```python
from build123d import *

# Parameters (mm, degrees)
SKETCH1_W           = 5
SKETCH1_H           = 5
BOSS_EXTRUDE1_DEPTH = 40
SKETCH2_W           = 51.86
SKETCH2_H           = 5
SKETCH2_W_2         = 5
BOSS_EXTRUDE3_DEPTH = 5
SKETCH4_W           = 25
SKETCH4_H           = 5
BOSS_EXTRUDE4_DEPTH = 15
FILLET1_R           = 1
FILLET2_R           = 1
FILLET3_R           = 1
SKETCH5_W           = 10
SKETCH5_H           = 6
CUT_EXTRUDE1_DEPTH  = 70.699782068


with BuildPart() as part:
    # Sketch1 → Boss-Extrude1 (new body)
    with BuildSketch(Plane(origin=(0, 0, 0), x_dir=(1, 0, 0), z_dir=(0, 1, 0))):
        with Locations((2.5, 2.5)):
            Rectangle(SKETCH1_W, SKETCH1_H)
    extrude(amount=BOSS_EXTRUDE1_DEPTH)

    # Sketch2 → Boss-Extrude3 (add)
    with BuildSketch(Plane.XZ):
        with Locations((30.93, -2.5)):
            Rectangle(SKETCH2_W, SKETCH2_H)
        with Locations((2.5, -2.5)):
            Rectangle(SKETCH2_W_2, SKETCH2_H)
    extrude(amount=BOSS_EXTRUDE3_DEPTH)

    # Sketch4 → Boss-Extrude4 (add)
    with BuildSketch(Plane.XZ.offset(5)):
        with Locations((44.36, -2.5)):
            Rectangle(SKETCH4_W, SKETCH4_H)
    extrude(amount=BOSS_EXTRUDE4_DEPTH)

    # Fillet1
    fillet1_edges = [part.edges().sort_by_distance(p)[0] for p in [
        (15.93, -5, 0),
        (56.86, -10, 0),
        (30.93, 0, 0),
        (31.86, -12.5, 0),
        (44.36, -20, 0),
    ]]
    fillet(fillet1_edges, radius=FILLET1_R)

    # Fillet2
    fillet2_edges = [part.edges().sort_by_distance(p)[0] for p in [
        (56.86, -10, -5),
        (30.93, 0, -5),
        (15.93, -5, -5),
        (31.86, -12.5, -5),
        (44.36, -20, -5),
    ]]
    fillet(fillet2_edges, radius=FILLET2_R)

    # Fillet3
    fillet3_edges = [part.edges().sort_by_distance(p)[0] for p in [
        (5, 0, -2.5),
        (5, -0.292893219, -0.292893219),
        (5, -0.292893219, -4.707106781),
    ]]
    fillet(fillet3_edges, radius=FILLET3_R)

    # Sketch5 → Cut-Extrude1 (cut, through all)
    with BuildSketch(Plane(origin=(0, 0, -5), x_dir=(-1, 0, 0), z_dir=(0, 0, -1))):
        with Locations((-45.36, -6.38)):
            Rectangle(SKETCH5_W, SKETCH5_H)
    extrude(amount=-CUT_EXTRUDE1_DEPTH, mode=Mode.SUBTRACT)


solid = part.part
```
Check sheet for the modelled part. Datum: model origin and axes. Units: mm. A direction names the side the tool comes from. Give positions to 0.01 mm unless a question says otherwise; leave off trailing zeros. Write each loop counter-clockwise with the first axis right and the second up, starting at its lowest first coordinate (ties: lowest second). Pieces come first, ordered by that corner, then holes. Notation, with made-up numbers: (-31, 52.25) -> (26, 52.25) arc R27 ccw to (26, 73.25) -> close; hole circle Ø7 at (-31.75, 36). An arc over 180 degrees is marked (long way). Use CSV: the item, a comma, the result in double quotes. Start each with the question number.
Q1. Cross-section at B-B on x = 45. Enter the section's corners in (y, z).
Q2. Tool access check on faces 1 (the flat face through (50.36, -6, -3)), 2 (the flat face through (28, -2, 0)), 3 (the flat face through (31.86, -12, -3)), 4 (the flat face through (31, 0, -2)). Record the directions out of +Z, -Z, +X, -X, +Y, -Y that give a thin tool (end or side, any length) a straight path to the whole face; none if there is none.
Q3. Cross-section at C-C on x = 7. Enter the section's corners in (y, z), and give its area (3 significant figures).
Q4. Depth check by flat-ended pin: P1, Ø1.5, axis at x = 33.5, z = -2.5, coming from the +Y side; P2, Ø3, axis at x = 8, z = -1.5, coming from the -Y side; P3, Ø0.9, axis at y = -16, z = -2.5, coming from the -X side. Enter the tip coordinate at first touch or a pass-through.
Q5. Cross-section at D-D on y = 21.5. Enter the section's corners in (x, z).
Q6. Scan lines: line 1 along Y through (x, z) = (46, -3.1); line 2 along X through (y, z) = (9, -1.8); line 3 along Y through (x, z) = (53, -3.6). Record each from-to range of solid material in increasing order.
Q7. Cross-section at A-A on z = -2.55. Enter the section's corners in (x, y), and give its area (3 significant figures).
Q8. Release check for a two-part mould opening along X. For faces 5 (the flat face through (56.86, -10, -3)), 6 (the flat face through (16, -5, -2)), 7 (the flat face through (45, -9.38, -3)), 8 (the flat face through (40.36, -6, -3)) record: +X half, -X half, draft (parallel to the pull), parting line (faces both ways), or undercut.
Working result:
1,outline,"(-20, -4) arc R1 ccw to (-19, -5) -> (-9.38, -5) -> (-9.38, 0) -> (-19, 0) arc R1 ccw to (-20, -1) -> close; (-3.38, -5) -> (-1, -5) arc R1 ccw to (0, -4) -> (0, -1) arc R1 ccw to (-1, 0) -> (-3.38, 0) -> close"
2,face 1,"+Z, -Z"
2,face 2,"+Z, +X, -X, +Y, -Y"
2,face 3,"+Z, -Z, -X, -Y"
2,face 4,"+Z, -Z, +X, +Y"
3,outline,"(-5, -4) arc R1 ccw to (-4, -5) -> (-1, -5) arc R1 ccw to (0, -4) -> (0, -1) arc R1 ccw to (-1, 0) -> (-4, 0) arc R1 ccw to (-5, -1) -> close"
3,area,"24.1 mm^2"
4,P1,"stops at y = 0"
4,P2,"stops at y = -5"
4,P3,"stops at x = 31.86"
5,outline,"(0, -5) -> (5, -5) -> (5, 0) -> (0, 0) -> close"
6,line 1,"y = -20 to -9.38, -3.38 to 0"
6,line 2,"x = 0 to 5"
6,line 3,"y = -20 to 0"
7,outline,"(0, -5) -> (31.86, -5) -> (31.86, -20) -> (56.86, -20) -> (56.86, 0) -> (6, 0) arc R1 cw to (5, 1) -> (5, 40) -> (0, 40) -> close; hole (40.36, -9.38) -> (50.36, -9.38) -> (50.36, -3.38) -> (40.36, -3.38) -> close"
7,area,"800 mm^2"
8,face 5,"+X half"
8,face 6,"draft"
8,face 7,"undercut"
8,face 8,"undercut"
